Design review of the part built by this model. Coordinates are the model's own, in mm. Face numbers are marked on the shaded views. Round coordinates to 2 decimals unless told otherwise and drop trailing zeros. Order: outer loops, then holes, each group sorted by start corner. A loop starts at its lowest first (then second) coordinate and runs counter-clockwise, first axis right, second up. Notation, with made-up numbers: (28.25, 34) - (45.25, 34) arc R24 ccw to (45.25, 52) - close; hole circle Ø9 at (48.25, -33.5). An arc over 180 degrees is marked (long way). Write item = value, one per line.
from build123d import *

# Parameters (mm, degrees)
F3_DEPTH  = 91.44
F6_R      = 4.2867636814
F7_DEPTH  = 76.2
F9_R      = 4.3700650399
F14_DEPTH = 29.972
F13_R     = 14.2738444306
F15_DEPTH = 21.59
F16_D     = 19.05
F16_DEPTH = 18.288
F16_TIP   = 5.7231973962


with BuildPart() as f3:
    # F0 (on Right) → F3 (new body)
    with BuildSketch(Plane.YZ):
        with BuildLine():
            ThreePointArc((0, 40.9521651562), (3.0523323842, 42.2164826266), (4.3166498546, 45.2688150108))
            ThreePointArc((4.3166498546, 45.2688150108), (3.0523323842, 48.321147395), (0, 49.5854648654))
            Line((0, 49.5854648654), (0, 40.9521651562))
        make_face()
        with BuildLine():
            Line((0, 40.9521651562), (0, 49.5854648654))
            ThreePointArc((0, 49.5854648654), (-4.3166498546, 45.2688150108), (0, 40.9521651562))
        make_face()
    extrude(amount=F3_DEPTH)



with BuildPart() as f4:
    # F0 (on Right) → F4 (revolve)
    with BuildSketch(Plane.YZ):
        with BuildLine():
            Line((0, 40.9521651562), (0, 49.5854648654))
            ThreePointArc((0, 49.5854648654), (-4.3166498546, 45.2688150108), (0, 40.9521651562))
        make_face()
    revolve(axis=Axis((0, 0, 45.2688150108), (0, 0, 1)))


with BuildPart() as f7:
    # F6 (on offset) → F7 (new body)
    with BuildSketch(Plane.XY.offset(45.26788)):
        Circle(F6_R)
    extrude(amount=-F7_DEPTH)


with BuildPart() as f8_1:
    # F8: copy of F4
    add(f4.part.moved(Location((0, 0, -76.2))))


with BuildPart() as f14:
    # F9 (on Right) → F14 (new body)
    with BuildSketch(Plane.YZ):
        with Locations((0.0073989029, -30.8914642022)):
            Circle(F9_R)
    extrude(amount=-F14_DEPTH)


with BuildPart() as f3_1:
    add(f3.part)

    add(f4.part)  # F15 merges F4

    add(f7.part)  # F15 merges F7

    add(f8_1.part)  # F15 merges F8_1

    add(f14.part)  # F15 merges F14
    # F13 (on offset) → F15 (join)
    with BuildSketch(Plane.YZ.offset(-29.972)):
        with Locations((0, -30.7933222502)):
            Circle(F13_R)
    extrude(amount=-F15_DEPTH)

    # F16
    with Locations(Plane(origin=(-51.562, 0, 0), x_dir=(0, 1, 0), z_dir=(-1, 0, 0))):
        with Locations((0, 30.8683142066)):
            Hole(F16_D / 2, depth=F16_DEPTH)
            with Locations((0, 0, -(F16_DEPTH + F16_TIP / 2))):  # 118° drill point
                Cone(0, F16_D / 2, F16_TIP, mode=Mode.SUBTRACT)


solid = f3_1.part
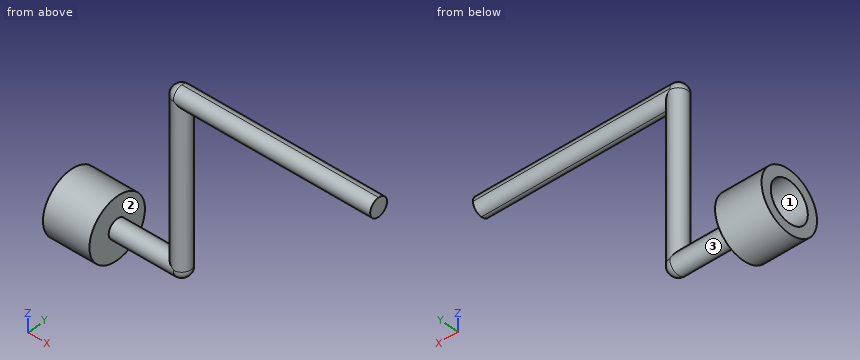
1) We need section B-B on x = 60.5. Write out the cut boundary in (y, z), and give its area (3 significant figures).
Findings:
outline = circle Ø8.63 at (0, 45.27)
area = 58.5 mm^2
2) We need section A-A on z = 37. Write out the cut boundary in (x, y), and give its area (3 significant figures).
Findings:
outline = circle Ø8.57 at (0, 0)
area = 57.7 mm^2
3) The part is to be moulded in two halves that separate along Z. For the marked faces 1, 2 and 3, say which applies: released by +Z, released by -Z, zero draft, split by the parting line, or undercut.
Findings:
face_1 = undercut
face_2 = zero draft
face_3 = split by the parting line
4) Clearance check with flat-ended pins moving along their axes: pin 1 Ø6 at (y, z) = (-1, -31.5) entering from +X; pin 2 Ø10 at (x, y) = (12.5, -11) entering from +Z; pin 3 Ø15 at (y, z) = (0, -30.87) entering from -X. State where each tip first meets the part, or that it passes through.
Findings:
pin_1 = 4.32
pin_2 = through
pin_3 = -32.06
5) To check wall thickness, follow L1, parallel to Z at x = -41.25, y = 0; L2, parallel to X at y = -7.75, z = -23.5; L3, parallel to Z at x = -29.5, y = 0.75. State the ranges of each line that lie inside material, in increasing order. Write a range as from..to.
Findings:
L1 = -45.07..-40.39, -21.34..-16.52
L2 = -51.56..-29.97
L3 = -35.2..-34.02, -27.71..-26.58
6) We need section C-C on y = -11.75. Write out the cut boundary in (x, z).
Findings:
outline = (-51.56, -38.9) - (-29.97, -38.9) - (-29.97, -22.69) - (-51.56, -22.69) - close
7) We need section D-D on x = -31.5. Write out the cut boundary in (y, z), and give its area (3 significant figures).
Findings:
outline = circle Ø28.55 at (0, -30.79); hole circle Ø13.15 at (0, -30.87)
area = 504 mm^2
